Design review of the part built by this model. Coordinates are the model's own, in mm. A direction names the side the tool comes from. Round coordinates to 2 decimals unless told otherwise and drop trailing zeros. Order: outer loops, then holes, each group sorted by start corner. A loop starts at its lowest first (then second) coordinate and runs counter-clockwise, first axis right, second up. Notation, with made-up numbers: (65, 8.5) - (88, 8.5) arc R34 cw to (88, 45.5) - close; hole circle Ø4 at (-30, -38). An arc over 180 degrees is marked (long way). Write item = value, one per line.
from build123d import *

# Parameters (mm, degrees)
F1_DEPTH = 6.35


with BuildPart() as f1:
    # F0 (on Front) → F1 (new body)
    with BuildSketch(Plane.XZ):
        with BuildLine():
            ThreePointArc((0, 11.0236), (-7.794862, -7.794862), (11.0236, 0))
            ThreePointArc((11.0236, 0), (7.794862, 7.794862), (0, 11.0236))
        make_face()
        with BuildLine():
            ThreePointArc((11.424853, 8.579359), (6.385729, 12.781045), (0, 14.2875))
            ThreePointArc((0, 14.2875), (-6.393397, 12.777211), (-11.435141, 8.565642))
            ThreePointArc((-11.435141, 8.565642), (-14.2875, 0), (-11.435141, -8.565642))
            ThreePointArc((-11.435141, -8.565642), (-0.008573, -14.287497), (11.424853, -8.579359))
            ThreePointArc((11.424853, -8.579359), (13.552956, -4.522172), (14.2875, 0))
            ThreePointArc((14.2875, 0), (13.552956, 4.522172), (11.424853, 8.579359))
        make_face()
        with BuildLine():
            ThreePointArc((0, 11.0236), (7.794862, 7.794862), (11.0236, 0))
            ThreePointArc((11.0236, 0), (-7.794862, -7.794862), (0, 11.0236))
        make_face(mode=Mode.SUBTRACT)
        with BuildLine():
            ThreePointArc((-11.435141, 8.565642), (-6.393397, 12.777211), (0, 14.2875))
            Line((0, 14.2875), (0, 15.382706))
            Line((0, 15.382706), (-0.010288, 15.376777))
            Line((-0.010288, 15.376777), (-11.435141, 21.984798))
            Line((-11.435141, 21.984798), (-11.435141, 8.565642))
        make_face()
        with BuildLine():
            Line((0, 15.382706), (0, 14.2875))
            ThreePointArc((0, 14.2875), (6.385729, 12.781045), (11.424853, 8.579359))
            Line((11.424853, 8.579359), (11.424853, 21.966979))
            Line((11.424853, 21.966979), (0, 15.382706))
        make_face()
        with BuildLine():
            Line((20.778073, 0), (11.424853, 8.579359))
            ThreePointArc((11.424853, 8.579359), (13.552956, 4.522172), (14.2875, 0))
            ThreePointArc((14.2875, 0), (13.552956, -4.522172), (11.424853, -8.579359))
            Line((11.424853, -8.579359), (20.778073, 0))
        make_face()
        with BuildLine():
            ThreePointArc((-11.435141, -8.565642), (-14.2875, 0), (-11.435141, 8.565642))
            Line((-11.435141, 8.565642), (-20.943042, 0))
            Line((-20.943042, 0), (-11.435141, -8.565642))
        make_face()
        Polygon((-0.005462, 18.48569), (0, 18.48884), (8.734868, 23.525615), (8.74033, 33.614925), (0.005462, 38.66431), (-8.734868, 33.624385), (-8.74033, 23.535075), align=None)
        Polygon((-0.010288, 15.376777), (0, 15.382706), (11.424853, 21.966979), (11.435141, 35.165202), (0.010288, 41.773223), (-11.424853, 35.183021), (-11.435141, 21.984798), align=None)
        Polygon((8.734868, 23.525615), (0, 18.48884), (-0.005462, 18.48569), (-8.74033, 23.535075), (-8.734868, 33.624385), (0.005462, 38.66431), (8.74033, 33.614925), align=None, mode=Mode.SUBTRACT)
        with BuildLine():
            ThreePointArc((11.424853, -8.579359), (-0.008573, -14.287497), (-11.435141, -8.565642))
            Line((-11.435141, -8.565642), (-11.435141, -21.965788))
            Line((-11.435141, -21.965788), (0, -15.375586))
            Line((0, -15.375586), (11.424853, -21.983607))
            Line((11.424853, -21.983607), (11.424853, -8.579359))
        make_face()
        Polygon((0, -15.375586), (-11.435141, -21.965788), (-11.445428, -35.164011), (-0.020576, -41.772032), (11.414565, -35.181831), (11.424853, -21.983607), align=None)
        Polygon((-0.004826, -18.484499), (8.730042, -23.533885), (8.72458, -33.623195), (-0.01575, -38.663119), (-8.750618, -33.613734), (-8.745156, -23.524424), align=None, mode=Mode.SUBTRACT)
    extrude(amount=F1_DEPTH)


solid = f1.part
1) We need section A-A on y = -4.5. Give the number of separate pieces and of enclosed holes in the cut face, and give its area (3 significant figures).
Findings:
separate_pieces = 1
enclosed_holes = 3
area = 1,010 mm^2
2) To check wall thickness, follow L1, parallel to X at y = -2.25, z = 31.5; L2, parallel to Z at x = -6, y = -1; L3, parallel to Z at x = 7, y = -4.25. State the ranges of each line that lie inside material, in increasing order. Write a range as from..to.
Findings:
L1 = -11.43..-8.74, 8.74..11.43
L2 = -38.31..-35.2, -21.94..-9.25, 9.25..21.95, 35.2..38.31
L3 = -37.73..-34.62, -22.53..-8.52, 8.52..22.53, 34.62..37.73
3) We need section D-D on z = -20. Write out the cut boundary in (x, y).
Findings:
outline = (-11.44, -6.35) - (-2.63, -6.35) - (-2.63, 0) - (-11.44, 0) - close; (2.62, -6.35) - (11.42, -6.35) - (11.42, 0) - (2.62, 0) - close
4) We need section C-C on x = -1. Write out the cut boundary in (y, z), and give its area (3 significant figures).
Findings:
outline = (-6.35, -41.21) - (0, -41.21) - (0, -38.09) - (-6.35, -38.09) - close; (-6.35, -19.06) - (0, -19.06) - (0, -10.98) - (-6.35, -10.98) - close; (-6.35, 10.98) - (0, 10.98) - (0, 19.06) - (-6.35, 19.06) - close; (-6.35, 38.08) - (0, 38.08) - (0, 41.19) - (-6.35, 41.19) - close
area = 142 mm^2
5) The part is to be moulded in two halves that separate along Z. For faces 1 (the flat face through (-4.426, -3.131, 36.109)), 2 (the flat face through (-16.123, -3.131, 4.343)), 3 (the flat face through (-5.813, -3.131, -38.422)), say which applies: released by +Z, released by -Z, zero draft, split by the parting line, or undercut.
Findings:
face_1 = undercut
face_2 = released by +Z
face_3 = released by -Z
6) Clearance check with flat-ended pins moving along their axes: pin 1 Ø1 at (x, y) = (-13, -5) entering from +Z; pin 2 Ø1.5 at (x, y) = (9.5, -4.5) entering from +Z; pin 3 Ø1.9 at (y, z) = (-3.5, 16.5) entering from -X. State where each tip first meets the part, or that it passes through.
Findings:
pin_1 = 7.61
pin_2 = 36.72
pin_3 = -11.44
7) For faces 4 (the flat face through (16.036, -3.131, -4.35)), 5 (the flat face through (4.416, -3.131, -36.108)), list the 3-axis set-ups (+Z, -Z, +X, -X, +Y, -Y) from which the entire face can be reached by the end or side of a thin tool; tool diameter is ignored.
Findings:
face_4 = -Z, +X, +Y, -Y
face_5 = +Y, -Y
8) We need section B-B on z = 5. Write out the cut boundary in (x, y).
Findings:
outline = (-15.39, -6.35) - (-9.82, -6.35) - (-9.82, 0) - (-15.39, 0) - close; (9.82, -6.35) - (15.33, -6.35) - (15.33, 0) - (9.82, 0) - close
